```python
from build123d import *

# Parameters (mm, degrees)
SKETCH1_W               = 40
SKETCH1_H               = 40
BOSS_EXTRUDE1_DEPTH     = 20
SKETCH2_R               = 5.6
CUT_EXTRUDE1_DEPTH      = 10
CHAMFER1_SIZE           = 1
F_1_4_20_TAPPED_HOLE1_D = 5.1054
SKETCH5_R               = 4
CUT_EXTRUDE2_DEPTH      = 41


with BuildPart() as part:
    # Sketch1 → Boss-Extrude1 (new body)
    with BuildSketch(Plane(origin=(0, 0, 0), x_dir=(1, 0, 0), z_dir=(0, 1, 0))):
        Rectangle(SKETCH1_W, SKETCH1_H)
    extrude(amount=BOSS_EXTRUDE1_DEPTH)

    # Sketch2 → Cut-Extrude1 (cut)
    with BuildSketch(Plane.ZY.offset(20)):
        with Locations((-10, 10)):
            Circle(SKETCH2_R)
    extrude(amount=-CUT_EXTRUDE1_DEPTH, mode=Mode.SUBTRACT)

    # Chamfer1
    chamfer1_edges = [part.edges().sort_by_distance(p)[0] for p in [
        (-20, 20, 0),
        (0, 20, 20),
        (20, 20, 0),
        (0, 0, 20),
        (-20, 0, 0),
        (0, 0, -20),
        (20, 0, 0),
        (0, 20, -20),
        (20, 10, 20),
        (-20, 10, 20),
        (-20, 10, -20),
        (20, 10, -20),
    ]]
    chamfer(chamfer1_edges, length=CHAMFER1_SIZE)

    # 1/4-20 Tapped Hole1 (through all)
    with Locations(Plane(origin=(0, 20, 0), x_dir=(1, 0, 0), z_dir=(0, 1, 0))):
        with Locations((15, -7.5), (15, 15)):
            Hole(F_1_4_20_TAPPED_HOLE1_D / 2)

    # Sketch5 → Cut-Extrude2 (cut, through all)
    with BuildSketch(Plane(origin=(0, 0, -20), x_dir=(-1, 0, 0), z_dir=(0, 0, -1))):
        with Locations((0, 10)):
            Circle(SKETCH5_R)
    extrude(amount=-CUT_EXTRUDE2_DEPTH, mode=Mode.SUBTRACT)


solid = part.part
```
Check sheet for the modelled part. Datum: model origin and axes. Units: mm. Round coordinates to 2 decimals unless told otherwise and drop trailing zeros. Order: outer loops, then holes, each group sorted by start corner. A loop starts at its lowest first (then second) coordinate and runs counter-clockwise, first axis right, second up. Notation, with made-up numbers: (-26.75, 39.5) - (-20.75, 39.5) arc R18 ccw to (-20.75, 74.5) - close; hole circle Ø9 at (59.5, 34.5). An arc over 180 degrees is marked (long way). Answer as CSV lines item,"result". Start each with the question number.
1) Section check B-B (y = 10). Record the cut outline in (x, z).
2) Section check A-A (x = 15). Record the cut outline in (y, z), then the cut area to 3 significant figures.
3) Section check C-C (z = 7.5). Record the cut outline in (x, y).
4) Draft check along Y on faces 1 (the face through (-19.5, 9.9, -19.5)), 2 (the face through (-15.07, 5.03, -7.42)), 3 (the face through (19.4, 0.7, -19.3)). Enter one of: +Y half, -Y half, draft (parallel to the pull), parting line (faces both ways), or undercut.
5) Depth check by flat-ended pin: pin 1 (6.5 mm diameter, centred on x = 15, z = -15, fed in from +Y); pin 2 (10 mm diameter, centred on y = 10, z = -10, fed in from -X); pin 3 (5 mm diameter, centred on x = 0, y = 10, fed in from +Z). Enter the tip coordinate at first touch or a pass-through.
6) Scan lines: probe 1 along Z at (x, y) = (15, 5); probe 2 along Z at (x, y) = (13.5, 2.75); probe 3 along X at (y, z) = (9.25, -14). Record each from-to range of solid material in increasing order.
7) Section check D-D (z = 14). Record the cut outline in (x, y).
Determined:
1,outline,"(-20, -19) - (-19, -20) - (-4, -20) - (-4, 20) - (-19, 20) - (-20, 19) - (-20, -4.4) - (-10, -4.4) - (-10, -15.6) - (-20, -15.6) - close; (4, -20) - (19, -20) - (20, -19) - (20, 19) - (19, 20) - (4, 20) - close; hole circle Ø5.11 at (15, -15); hole circle Ø5.11 at (15, 7.5)"
2,outline,"(0, -19) - (1, -20) - (19, -20) - (20, -19) - (20, -17.55) - (0, -17.55) - close; (0, -12.45) - (20, -12.45) - (20, 4.95) - (0, 4.95) - close; (0, 10.05) - (20, 10.05) - (20, 19) - (19, 20) - (1, 20) - (0, 19) - close"
2,area,"594 mm^2"
3,outline,"(-20, 1) - (-19, 0) - (12.45, 0) - (12.45, 20) - (-19, 20) - (-20, 19) - close; (17.55, 0) - (19, 0) - (20, 1) - (20, 19) - (19, 20) - (17.55, 20) - close; hole circle Ø8 at (0, 10)"
4,face 1,"draft"
4,face 2,"undercut"
4,face 3,"-Y half"
5,pin 1,"y = 20"
5,pin 2,"x = -10"
5,pin 3,"through"
6,probe 1,"-20 to -17.55, -12.45 to 4.95, 10.05 to 20"
6,probe 2,"-20 to -17.07, -12.93 to 5.43, 9.57 to 20"
6,probe 3,"-10 to -3.93, 3.93 to 12.65, 17.35 to 20"
7,outline,"(-20, 1) - (-19, 0) - (19, 0) - (20, 1) - (20, 19) - (19, 20) - (-19, 20) - (-20, 19) - close; hole circle Ø8 at (0, 10)"
